Geometry check sheet. Reference: drawing and pictorial views, mm from the part's lowest x, y, z. Give positions to 0.01 mm unless a question says otherwise; leave off trailing zeros. Order: outer loops, then holes, each group sorted by start corner. A loop starts at its lowest first (then second) coordinate and runs counter-clockwise, first axis right, second up.
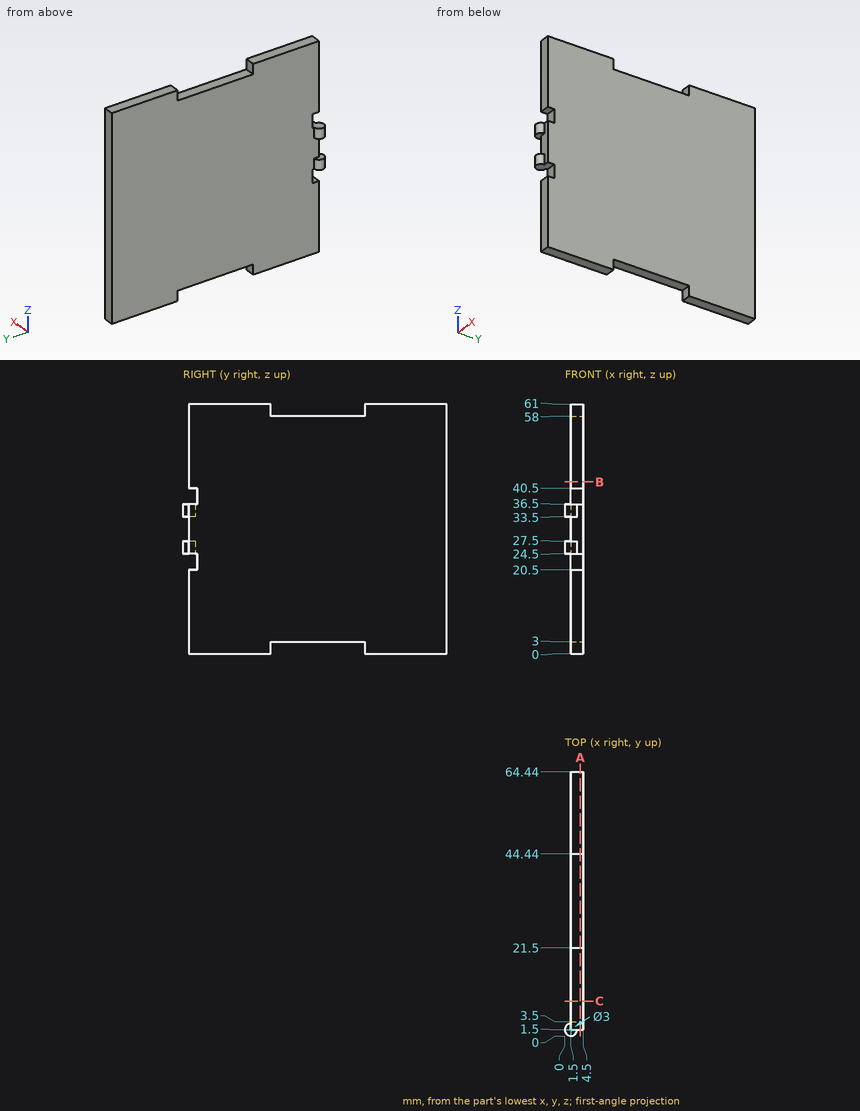
1) Material ranges on L1, parallel to Z at x = 3.55, y = 31.5; L2, parallel to X at y = 35, z = 33; L3, parallel to Y at x = 3.25, z = 28.5, recorded low to high.
Recorded:
L1: z = 3 to 58
L2: x = 1.5 to 4.5
L3: y = 1.5 to 64.44
2) Section check C-C, the plane y = 8.5. Record the cut outline in (x, z), then the cut area to 3 significant figures.
Recorded:
outline: (1.5, 0) - (4.5, 0) - (4.5, 61) - (1.5, 61) - close
area: 183 mm2
3) Section check B-B, the plane z = 42. Record the cut outline in (x, y), then the cut area to 3 significant figures.
Recorded:
outline: (1.5, 1.5) - (4.5, 1.5) - (4.5, 64.44) - (1.5, 64.44) - close
area: 189 mm2
4) Depth check by flat-ended pin: pin 1 Ø2.5 at (x, y) = (3.5, 37) entering from -Z; pin 2 Ø2.5 at (x, z) = (2.5, 21.5) entering from -Y; pin 3 Ø12 at (y, z) = (35.5, 10) entering from -X. Enter the tip coordinate at first touch or a pass-through.
Recorded:
pin 1: stops at z = 3
pin 2: stops at y = 1.5
pin 3: stops at x = 1.5
5) Section check A-A, the plane x = 3.8. Record the cut outline in (y, z).
Recorded:
outline: (1.5, 0) - (21.5, 0) - (21.5, 3) - (44.44, 3) - (44.44, 0) - (64.44, 0) - (64.44, 61) - (44.44, 61) - (44.44, 58) - (21.5, 58) - (21.5, 61) - (1.5, 61) - (1.5, 40.5) - (3.5, 40.5) - (3.5, 36.5) - (1.5, 36.5) - (1.5, 24.5) - (3.5, 24.5) - (3.5, 20.5) - (1.5, 20.5) - close
